Input: dimensioned drawing with shaded views. Units: mm. Origin: part minimum x, y, z. A direction names the side the tool comes from. Round coordinates to 2 decimals unless told otherwise and drop trailing zeros. Order: outer loops, then holes, each group sorted by start corner. A loop starts at its lowest first (then second) coordinate and runs counter-clockwise, first axis right, second up. Notation, with made-up numbers: (3.25, -9.75) - (7.25, -9.75) arc R28 ccw to (7.25, 18.25) - close; hole circle Ø10 at (-34, -18.5). An arc over 180 degrees is marked (long way). Put each result on its own line as item: value. Start each with the question number.
(1) Pin query (flat end, axial travel): P1, Ø1.5, axis at y = 1, z = 7.5, coming from the -X side; P2, Ø1.3, axis at x = 9, y = 1, coming from the +Z side. Return the tip coordinate at first contact, or that it passes through.
(2) Material intervals for L1, parallel to Z at x = 6, y = 1.7; L2, parallel to X at y = 0.75, z = 11 (1 decimal); L3, parallel to X at y = 2.4, z = 0.75 (1 decimal), sorted ascending. Write a range as [from, to].
(3) Section C-C (x = 5.5). Output: boundary loops of the cut face in (y, z).
(4) Access query for the marked faces 1 and 2. Directions: +Z, -Z, +X, -X, +Y, -Y. A direction counts if a zero-diameter tool reaches every point of the face in a straight line with its end or side. Return the directions, or none.
(5) Section A-A (y = 2.1). Output: boundary loops of the cut face in (x, z) (1 decimal).
(6) Section B-B (z = 7.25). Output: boundary loops of the cut face in (x, y) (1 decimal).
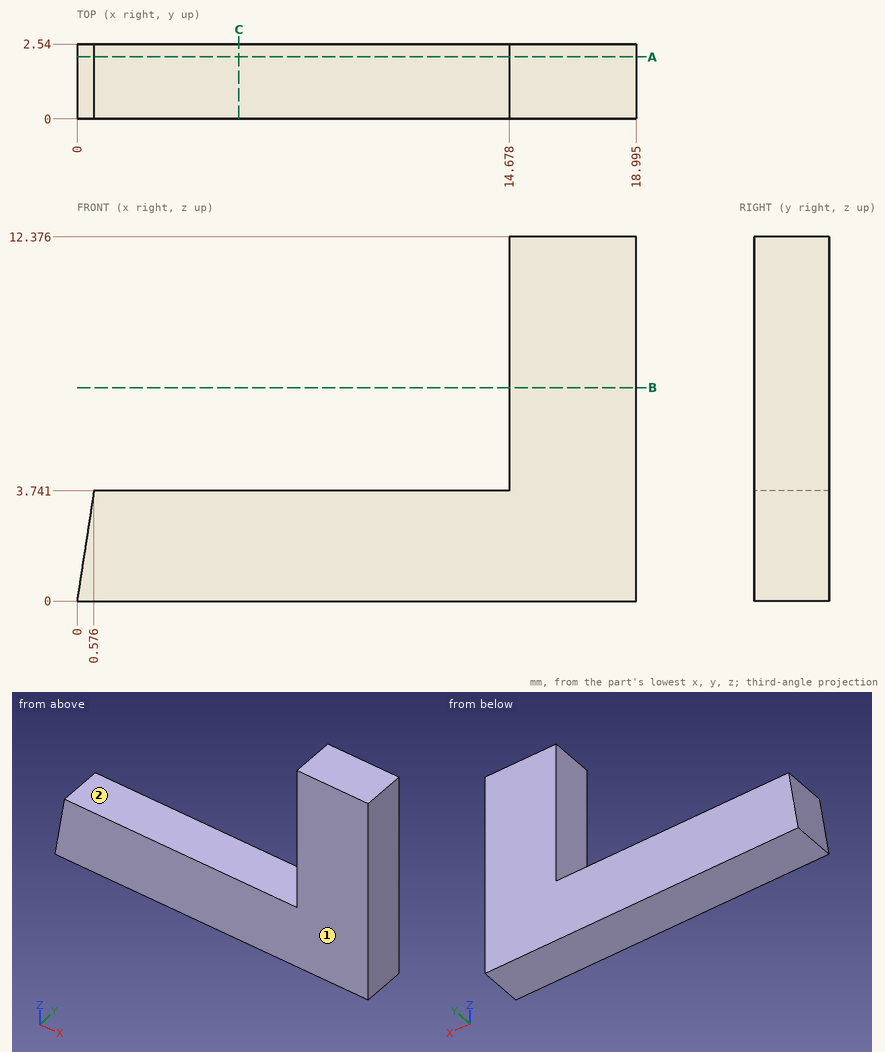
Checks:
1. P1: stops at x = 14.68
1. P2: stops at z = 3.74
2. L1: z = [0, 3.74]
2. L2: x = [14.7, 19]
2. L3: x = [0.1, 19]
3. outline: (0, 0) - (2.54, 0) - (2.54, 3.74) - (0, 3.74) - close
4. face 1: +Z, -Z, +X, -X, -Y
4. face 2: +Z, -X, +Y, -Y
5. outline: (0, 0) - (19, 0) - (19, 12.4) - (14.7, 12.4) - (14.7, 3.7) - (0.6, 3.7) - close
6. outline: (14.7, 0) - (19, 0) - (19, 2.5) - (14.7, 2.5) - close
